from build123d import *

# Parameters (mm, degrees)
F1_DEPTH = 40.513
F2_DEPTH = 38.1
F3_DEPTH = 64.77
F5_R     = 5.08
F6_R     = 0.762


with BuildPart() as f1:
    # F0 (on Front) → F1 (new body)
    with BuildSketch(Plane.XZ):
        with BuildLine():
            Line((8.89, 22.7287972945), (8.89, 24.5818064272))
            Line((8.89, 24.5818064272), (3.5665511583, 24.5818064272))
            ThreePointArc((3.5665511583, 24.5818064272), (6.2968108914, 23.8521946995), (8.89, 22.7287972945))
        make_face()
        with BuildLine():
            Line((3.5665511583, 24.5818064272), (8.89, 24.5818064272))
            ThreePointArc((8.89, 24.5818064272), (0, 27.4567800376), (-8.89, 24.5818064272))
            Line((-8.89, 24.5818064272), (-3.5665511583, 24.5818064272))
            ThreePointArc((-3.5665511583, 24.5818064272), (0, 24.9167800376), (3.5665511583, 24.5818064272))
        make_face()
        with BuildLine():
            ThreePointArc((8.89, 22.7287972945), (6.2968108914, 23.8521946995), (3.5665511583, 24.5818064272))
            Line((3.5665511583, 24.5818064272), (-3.5665511583, 24.5818064272))
            ThreePointArc((-3.5665511583, 24.5818064272), (-6.2968108914, 23.8521946995), (-8.89, 22.7287972945))
            Line((-8.89, 22.7287972945), (8.89, 22.7287972945))
        make_face()
        with BuildLine():
            Line((-3.5665511583, 24.5818064272), (3.5665511583, 24.5818064272))
            ThreePointArc((3.5665511583, 24.5818064272), (0, 24.9167800376), (-3.5665511583, 24.5818064272))
        make_face()
        with BuildLine():
            Line((8.89, -3.4254523647), (8.89, 22.7287972945))
            Line((8.89, 22.7287972945), (-8.89, 22.7287972945))
            Line((-8.89, 22.7287972945), (-8.89, -3.4254523647))
            ThreePointArc((-8.89, -3.4254523647), (-8.4916458882, -5.2919635487), (-7.366, -6.8332199624))
            Line((-7.366, -6.8332199624), (-4.953, -6.8332199624))
            Line((-4.953, -6.8332199624), (-4.953, -4.1093734175))
            Line((-4.953, -4.1093734175), (-4.953, 0))
            Line((-4.953, 0), (-4.953, 6.8332199624))
            Line((-4.953, 6.8332199624), (4.953, 6.8332199624))
            Line((4.953, 6.8332199624), (4.953, 0))
            Line((4.953, 0), (4.953, -4.1093734175))
            Line((4.953, -4.1093734175), (4.953, -6.8332199624))
            Line((4.953, -6.8332199624), (7.366, -6.8332199624))
            ThreePointArc((7.366, -6.8332199624), (8.4916458882, -5.2919635487), (8.89, -3.4254523647))
        make_face()
        with BuildLine():
            Line((-3.5665511583, 24.5818064272), (-8.89, 24.5818064272))
            Line((-8.89, 24.5818064272), (-8.89, 22.7287972945))
            ThreePointArc((-8.89, 22.7287972945), (-6.2968108914, 23.8521946995), (-3.5665511583, 24.5818064272))
        make_face()
        with BuildLine():
            Line((3.683, -6.8332199624), (4.953, -6.8332199624))
            Line((4.953, -6.8332199624), (4.953, -4.1093734175))
            ThreePointArc((4.953, -4.1093734175), (4.6198986953, -5.6120576825), (3.683, -6.8332199624))
        make_face()
        with BuildLine():
            Line((-3.683, -6.8332199624), (3.683, -6.8332199624))
            ThreePointArc((3.683, -6.8332199624), (4.6198986953, -5.6120576825), (4.953, -4.1093734175))
            Line((4.953, -4.1093734175), (4.953, 0))
            ThreePointArc((4.953, 0), (0, -4.953), (-4.953, 0))
            Line((-4.953, 0), (-4.953, -4.1093734175))
            ThreePointArc((-4.953, -4.1093734175), (-4.6198986953, -5.6120576825), (-3.683, -6.8332199624))
        make_face()
        with BuildLine():
            Line((-4.953, -4.1093734175), (-4.953, -6.8332199624))
            Line((-4.953, -6.8332199624), (-3.683, -6.8332199624))
            ThreePointArc((-3.683, -6.8332199624), (-4.6198986953, -5.6120576825), (-4.953, -4.1093734175))
        make_face()
        with BuildLine():
            ThreePointArc((-4.953, 0), (0, -4.953), (4.953, 0))
            ThreePointArc((4.953, 0), (0, 4.953), (-4.953, 0))
        make_face()
        with BuildLine():
            ThreePointArc((-4.953, 0), (0, 4.953), (4.953, 0))
            Line((4.953, 0), (4.953, 6.8332199624))
            Line((4.953, 6.8332199624), (-4.953, 6.8332199624))
            Line((-4.953, 6.8332199624), (-4.953, 0))
        make_face()
    extrude(amount=F1_DEPTH)

    # F0 (on Front) → F2 (cut)
    with BuildSketch(Plane.XZ):
        with BuildLine():
            Line((-3.5665511583, 24.5818064272), (-8.89, 24.5818064272))
            Line((-8.89, 24.5818064272), (-8.89, 22.7287972945))
            ThreePointArc((-8.89, 22.7287972945), (-6.2968108914, 23.8521946995), (-3.5665511583, 24.5818064272))
        make_face()
        with BuildLine():
            Line((3.5665511583, 24.5818064272), (8.89, 24.5818064272))
            ThreePointArc((8.89, 24.5818064272), (0, 27.4567800376), (-8.89, 24.5818064272))
            Line((-8.89, 24.5818064272), (-3.5665511583, 24.5818064272))
            ThreePointArc((-3.5665511583, 24.5818064272), (0, 24.9167800376), (3.5665511583, 24.5818064272))
        make_face()
        with BuildLine():
            Line((8.89, 22.7287972945), (8.89, 24.5818064272))
            Line((8.89, 24.5818064272), (3.5665511583, 24.5818064272))
            ThreePointArc((3.5665511583, 24.5818064272), (6.2968108914, 23.8521946995), (8.89, 22.7287972945))
        make_face()
    extrude(amount=F2_DEPTH, mode=Mode.SUBTRACT)

    # F0 (on Front) → F3 (join)
    with BuildSketch(Plane.XZ):
        with BuildLine():
            Line((-3.683, -6.8332199624), (3.683, -6.8332199624))
            ThreePointArc((3.683, -6.8332199624), (4.6198986953, -5.6120576825), (4.953, -4.1093734175))
            Line((4.953, -4.1093734175), (4.953, 0))
            ThreePointArc((4.953, 0), (0, -4.953), (-4.953, 0))
            Line((-4.953, 0), (-4.953, -4.1093734175))
            ThreePointArc((-4.953, -4.1093734175), (-4.6198986953, -5.6120576825), (-3.683, -6.8332199624))
        make_face()
        with BuildLine():
            ThreePointArc((-4.953, 0), (0, -4.953), (4.953, 0))
            ThreePointArc((4.953, 0), (0, 4.953), (-4.953, 0))
        make_face()
        with BuildLine():
            ThreePointArc((-4.953, 0), (0, 4.953), (4.953, 0))
            Line((4.953, 0), (4.953, 6.8332199624))
            Line((4.953, 6.8332199624), (-4.953, 6.8332199624))
            Line((-4.953, 6.8332199624), (-4.953, 0))
        make_face()
    extrude(amount=F3_DEPTH)

    # F4: F1 across plane


with BuildPart() as f1_1:
    add(f1.part)
    add(f1.part.mirror(Plane.XZ))

    # F5
    f5_edges = [f1_1.edges().sort_by_distance(p)[0] for p in [
        (0, -40.513, 6.83322),
        (0, 40.513, 6.83322),
    ]]
    fillet(f5_edges, radius=F5_R)

    # F6
    f6_edges = [f1_1.edges().sort_by_distance(p)[0] for p in [
        (-4.953, 40.513, 1.361923),
        (-4.619899, 40.513, -5.612058),
        (-4.953, -40.513, 1.361923),
        (-4.619899, -40.513, -5.612058),
        (4.619899, -40.513, -5.612058),
        (4.953, -40.513, 1.361923),
        (4.953, 40.513, 1.361923),
        (4.619899, 40.513, -5.612058),
        (-4.953, 40.513, 9.37322),
        (4.953, 40.513, 9.37322),
        (-4.953, -40.513, 9.37322),
        (4.953, -40.513, 9.37322),
    ]]
    fillet(f6_edges, radius=F6_R)


solid = f1_1.part
The model under review builds one solid part; all positions refer to its coordinate system, in mm. A direction names the side the tool comes from. Round coordinates to 2 decimals unless told otherwise and drop trailing zeros. Order: outer loops, then holes, each group sorted by start corner. A loop starts at its lowest first (then second) coordinate and runs counter-clockwise, first axis right, second up. Notation, with made-up numbers: (-18.5, 36.25) -> (7.5, 36.25) arc R11 cw to (7.5, 55.25) -> close; hole circle Ø4 at (73.25, 78.5). An arc over 180 degrees is marked (long way). Use CSV: the item, a comma, the result in double quotes. Start each with the question number.
(1) Mouldability with a two-part tool opening along Y and no side actions: class faces 5 (the face through (0, 40.513, 14)), 6 (the face through (0, -38.1, 26)), 7 (the face through (0.133, 39.29, 27.456)) as pulls with the +Y half, pulls with the -Y half, needs draft (parallel to the pull), parting line crosses it, or undercut.
(2) Insertion check: pin 1 (10.5 mm diameter, centred on y = -50, z = 4, fed in from -X); pin 2 (5 mm diameter, centred on x = 1.5, z = 24, fed in from -Y); pin 3 (3 mm diameter, centred on x = 0.5, y = -59, fed in from +Z). Each pin has a flat end and moves straight along its axis. Give the tip position at first contact, or say it passes through.
(3) Consider section D-D on y = 49. Write out the cut boundary in (x, z), and give its area (3 significant figures).
(4) Consider section C-C on x = -1. Write out the cut boundary in (y, z).
(5) Consider section A-A on z = 3. Write out the cut boundary in (x, y) (3 decimals), and give its area (3 significant figures).
(6) Wall thickness on probe 1 along X at (y, z) = (-43.5, 4.5); probe 2 along Y at (x, z) = (4, 20.5); probe 3 along Z at (x, y) = (1.75, 55.5): over which ranges is each line inside the solid? List them lowest first. Write a range as from..to.
(7) Tool access review of faces 1 (the face through (4.61, 52.86, -5.63)), 2 (the face through (4.953, 53, 1)), 3 (the face through (0, 38.1, 26)), 4 (the face through (-4.63, 52.86, -5.59)): name each direction out of +Z, -Z, +X, -X, +Y, -Y from which nothing blocks a thin tool from reaching the whole face with its end or side.
(8) Consider section B-B on y = 22.5. Write out the cut boundary in (x, z).
Responses:
1,face 5,"pulls with the +Y half"
1,face 6,"undercut"
1,face 7,"needs draft"
2,pin 1,"x = -4.95"
2,pin 2,"y = -40.51"
2,pin 3,"z = 6.83"
3,outline,"(-4.95, -4.11) arc R3.56 ccw to (-3.68, -6.83) -> (3.68, -6.83) arc R3.56 ccw to (4.95, -4.11) -> (4.95, 6.83) -> (-4.95, 6.83) -> close"
3,area,"133 mm²"
4,outline,"(-64.77, -6.83) -> (64.77, -6.83) -> (64.77, 6.83) -> (45.59, 6.83) arc R5.08 cw to (40.51, 11.91) -> (40.51, 27.42) -> (38.1, 27.42) -> (38.1, 24.89) -> (-38.1, 24.89) -> (-38.1, 27.42) -> (-40.51, 27.42) -> (-40.51, 11.91) arc R5.08 cw to (-45.59, 6.83) -> (-64.77, 6.83) -> close"
5,outline,"(-8.89, -40.513) -> (-5.715, -40.513) arc R0.762 cw to (-4.953, -41.275) -> (-4.953, -64.77) -> (4.953, -64.77) -> (4.953, -41.275) arc R0.762 cw to (5.715, -40.513) -> (8.89, -40.513) -> (8.89, 40.513) -> (5.715, 40.513) arc R0.762 cw to (4.953, 41.275) -> (4.953, 64.77) -> (-4.953, 64.77) -> (-4.953, 41.275) arc R0.762 cw to (-5.715, 40.513) -> (-8.89, 40.513) -> close"
5,area,"1,920 mm²"
6,probe 1,"-4.95..4.95"
6,probe 2,"-40.51..40.51"
6,probe 3,"-6.83..6.83"
7,face 1,"-Z, +X, +Y"
7,face 2,"+Z, -Z, +X, +Y"
7,face 3,"+Z"
7,face 4,"-Z, -X, +Y"
8,outline,"(-8.89, -3.43) arc R4.57 ccw to (-7.37, -6.83) -> (7.37, -6.83) arc R4.57 ccw to (8.89, -3.43) -> (8.89, 22.73) arc R19.15 ccw to (-8.89, 22.73) -> close"
